Geometry check sheet. Reference: the model listing, model coordinates, mm. A direction names the side the tool comes from. Coordinates: 2 decimals unless noted, no trailing zeros. Order: outer loops, then holes, each group sorted by start corner. A loop starts at its lowest first (then second) coordinate and runs counter-clockwise, first axis right, second up. Notation, with made-up numbers: M -8,9.5 L 34,9.5 A9 cw 34,13.5 Z; hole C -18,81 d8. An arc over 180 degrees is marked long. One line per item, written item: value. Start each with the question number.
1) Sectioned sample at A-A, the plane z = 16. Enter the section's corners in (x, y).
2) Go/stop test with flat-tipped pins: P1, Ø12, axis at x = 10, z = 7, coming from the +Y side; P2, Ø12, axis at x = -21.5, z = 21, coming from the -Y side; P3, Ø3, axis at y = -8, z = -1, coming from the -X side. Record where each tip stops, or that it passes through.
3) Sectioned sample at C-C, the plane x = 0. Enter the section's corners in (y, z), then the cut area to 3 significant figures.
4) Draft check along Z on faces 1 (the flat face through (0, -25, 0)), 2 (the cylindrical face through (12.68, 1.35, -12.96)), 3 (the cylindrical face through (12.4, 1.4, 13.3)), 4 (the cylindrical face through (0.52, 1.87, -27.44)). Enter one of: pulls with the +Z half, pulls with the -Z half, needs draft (parallel to the pull), parting line crosses it, or undercut.
5) Sectioned sample at B-B, the plane x = 16.5. Enter the section's corners in (y, z).
6) Access from +Z, -Z, +X, -X, +Y, -Y to the whole of each face (thin tool, end or side, straight path). Record for faces 5 (the cylindrical face through (-13.581, 1.351, -12.206)), 6 (the cylindrical face through (-0.59, -12.32, -4.46)).
7) Thickness scan on L1, parallel to Z at x = -16, y = 2.85; L2, parallel to Y at x = 26, z = 9.5; L3, parallel to Y at x = -10.5, z = -28. Record the ranges inside material, lowest first. Write a range as from..to.
8) Sectioned sample at D-D, the plane y = -7.5. Enter the section's corners in (x, z).
Autodesk Inventor part; units mm, degrees
ref_plane "YZ Plane" through (0, 0, 0) normal (1, 0, 0) x (0, 1, 0)
ref_plane "XZ Plane" through (0, 0, 0) normal (0, 1, 0) x (-1, 0, 0)
ref_plane "XY Plane" through (0, 0, 0) normal (0, 0, 1) x (1, 0, 0)
sketch "Sketch1" plane through (0, 0, 0) normal (0, 1, 0) x (-1, 0, 0)
  line L0 (37.5, -37.5) -> (-37.5, -37.5)
  line L1 (-37.5, -37.5) -> (-37.5, 37.5)
  line L2 (-37.5, 37.5) -> (37.5, 37.5)
  line L3 (37.5, 37.5) -> (37.5, -37.5)
  line L4 (37.5, -37.5) -> (-37.5, 37.5) construction
  line L5 (-37.5, -37.5) -> (37.5, 37.5) construction
  point P0 (0, 0)
  dimension "d0" = 75
  dimension "d1" = 75
sketch "Sketch2" plane through (0, 0, 0) normal (0, 1, 0) x (-1, 0, 0)
  line L0 (-25, -25) -> (25, -25)
  line L1 (25, -25) -> (25, 25)
  line L2 (25, 25) -> (-25, 25)
  line L3 (-25, 25) -> (-25, -25)
  line L4 (-25, -25) -> (25, 25) construction
  line L5 (25, -25) -> (-25, 25) construction
  point P0 (0, 0)
  dimension "d2" = 50
  dimension "d3" = 50
extrude "Extrusion1" add sketch "Sketch1" along normal blind 4
extrude "Extrusion2" [suppressed]
sketch "Sketch3" plane through (37.5, 0, 37.5) normal (1, 0, 0) x (0, 0, -1)
  line L0 (75, 4) -> (0, 4)
  line L1 (0, 0) -> (75, 0)
  line L2 (0, 0) -> (75, 0)
  arc A0 (75, 0) -> (0, 0) centre (37.5, -173.7812) ccw
  point P0 (37.5, 4)
extrude "Extrusion3" cut sketch "Sketch3" against normal through all keep common part
sketch "Sketch4" plane through (37.5, 0, -37.5) normal (0, 0, -1) x (-1, 0, 0)
  line L0 (75, 0) -> (75, 4)
  line L1 (0, 0) -> (75, 0)
  line L2 (0, 0) -> (0, 4)
  line L3 (75, 0) -> (0, 0)
  arc A0 (75, 0) -> (0, 0) centre (37.5, -173.7813) ccw
  point P0 (37.5, 0)
extrude "Extrusion4" cut sketch "Sketch4" against normal through all keep common part
sketch "Sketch5" plane through (0, 0, 0) normal (0, -1, 0) x (1, 0, 0)
  circle A0 centre (0, 0) radius 4.5
  dimension "d14" = 9
extrude "Extrusion5" add sketch "Sketch5" along normal blind 25
sketch "Sketch6" plane through (0, 0, 0) normal (0, -1, 0) x (1, 0, 0)
  circle A0 centre (-16, -16) radius 4.5
  circle A1 centre (16, 16) radius 4.5
  line L0 (0, 0) -> (37.5, 37.5)
  circle A2 centre (16, -16) radius 4.5
  circle A3 centre (-16, 16) radius 4.5
  point P0 (0, 0)
  dimension "d17" = 9
  dimension "d18" = 9
  dimension "d19" = 16
  dimension "d20" = 16
  dimension "d21" = 16
  dimension "d22" = 16
  dimension "d25" = 9
  dimension "d26" = 9
extrude "Extrusion6" cut sketch "Sketch6" against normal through all
properties part number "thumper-bumper-trigger"
Final values:
1. outline: M -37.5,0 L -20.5,0 L -20.5,2.81 A177.78 ccw Z; M -11.5,0 L 11.5,0 L 11.5,3.28 L -11.5,3.28 Z; M 20.5,0 L 37.5,0 A177.78 ccw 20.5,2.81 Z
2. P1: stops at y = 3.94
2. P2: stops at y = 0
2. P3: stops at x = -4.5
3. outline: M -25,-4.5 L 0,-4.5 L 0,-37.5 A177.78 ccw 4,-0.03 L 4,0.03 A177.78 ccw 0,37.5 L 0,4.5 L -25,4.5 Z
3. area: 425 mm^2
4. face 1: needs draft
4. face 2: undercut
4. face 3: undercut
4. face 4: pulls with the -Z half
5. outline: M 0,-37.5 A177.78 ccw 2.82,-20.47 L 0,-20.47 Z; M 0,-11.53 L 3.23,-11.53 L 3.23,11.53 L 0,11.53 Z; M 0,20.47 L 2.82,20.47 A177.78 ccw 0,37.5 Z
6. face 5: +Y, -Y
6. face 6: -Y
7. L1: z = -11.5..11.5
7. L2: y = 0..2.09
7. L3: y = 0..1.78
8. outline: C 0,0 d9
